Autodesk Inventor part; units mm, degrees
ref_plane "YZ Plane" through (0, 0, 0) normal (1, 0, 0) x (0, 1, 0)
ref_plane "XZ Plane" through (0, 0, 0) normal (0, 1, 0) x (-1, 0, 0)
ref_plane "XY Plane" through (0, 0, 0) normal (0, 0, 1) x (1, 0, 0)
sketch "スケッチ1" plane through (0, 0, 0) normal (0, 0, 1) x (1, 0, 0)
  line L0 (8.5, 7) -> (-8.5, 7)
  line L1 (-8.5, 7) -> (-8.5, -7)
  line L2 (-8.5, -7) -> (8.5, -7)
  line L3 (8.5, -7) -> (8.5, 7)
  line L4 (8.5, 7) -> (-8.5, -7) construction
  line L5 (-8.5, 7) -> (8.5, -7) construction
  circle A0 centre (-6, 0) radius 1.5
  circle A1 centre (6, 0) radius 1.5
  line L6 (-8.5, -6) -> (8.5, -6)
  line L7 (-8.5, 4.5) -> (8.5, 4.5)
  line L8 (-4, -7) -> (-4, 7)
  line L9 (4, -7) -> (4, 7)
  line L10 (2.5, -6) -> (2.5, 4.5)
  line L11 (-2.5, -6) -> (-2.5, 4.5)
  line L12 (1.8, -6) -> (1.8, 4.5)
  line L13 (-1.8, -6) -> (-1.8, 4.5)
  point P0 (0, 0)
  point P1 (-4, -6)
  point P2 (-4, 4.5)
  point P3 (4, -6)
  point P4 (4, 4.5)
  dimension "d0" = 17
  dimension "d1" = 14
  dimension "d2" = 3
  dimension "d3" = 3
  dimension "d4" = 2.5
  dimension "d5" = 4.5
  dimension "d6" = 4.5
  dimension "d7" = 1.5
  dimension "d8" = 1.5
  dimension "d9" = 1
  dimension "d16" = 0.7
  dimension "d17" = 0.7
extrude "押し出し1" add sketch "スケッチ1" along normal blind 7 contours L3 L7 L9 L0 | L9 L7 L8 L0 | L3 L6 L9 L7 | L8 L7 L1 L0 | L3 L2 L9 L6 | L8 L6 L1 L7 | L10 L6 L12 L7 | L9 L2 L8 L6 | L7 L13 L6 L11 | L8 L2 L1 L6
sketch "スケッチ2" plane through (0, 0, 7) normal (0, 0, 1) x (1, 0, 0)
  line L0 (8.5, 7) -> (-8.5, 7)
  line L1 (0, 7) -> (-4, 7)
  line L2 (-4, 7) -> (-4, -7)
  line L3 (-8.5, -7) -> (8.5, -7)
  line L4 (-4, -7) -> (4, -7)
  line L5 (4, -7) -> (4, 7)
  line L6 (4, 7) -> (0, 7)
  point P0 (0, 0)
  dimension "d12" = 4
  dimension "d13" = 8
extrude "押し出し2" cut sketch "スケッチ2" against normal blind 0.6
properties part number "greiper_TPU" material "ゴム、シリコーン"
Model file for the job. Use its own axes, mm. A direction names the side the tool comes from. Coordinates: 2 decimals unless noted, no trailing zeros. Loops run counter-clockwise (first coordinate to the right, second up) from the corner with the lowest first, then second, coordinate; pieces in that order, holes last. Notation, with made-up numbers: (48.5, 6.25) - (95.5, 6.25) arc R31 ccw to (95.5, 37.25) - close; hole circle Ø11 at (-35.5, 2). An arc over 180 degrees is marked (long way). Answer as a JSON object with one key per item and string values. Group by question number.
(1) Cut at D-D (y = -2.5). Give the cut face in (x, z).
(2) Probe line 1 along X through (y, z) = (-3.5, 5.75); line 2 along Y through (x, z) = (-3.5, 5); line 3 along Y through (x, z) = (6, 5.75). List the from-to ranges inside material, lowest first.
(3) Two-plate mould, pull along X, no slides. Class faces 1 (the face through (-3, 4.5, 3)), 2 (the face through (-2.5, -1, 3)), 3 (the face through (-8.5, 0, 3)), 4 (the face through (8, 0, 7)): released by +X, released by -X, zero draft, split by the parting line, or undercut.
(4) Cut at A-A (x = 3.5). Give the cut face in (y, z), then the cut area to 3 significant figures.
(5) Tool access for faces 5 (the face through (0, -6, 3)), 6 (the face through (-2, 2, 6.4)), 7 (the face through (-8, 0, 7)): list every direction of +Z, -Z, +X, -X, +Y, -Y with a clear straight run to the whole face (end or side of a thin tool).
(6) Cut at C-C (z = 5.5). Give the cut face in (x, y), then the cut area to 3 significant figures.
(7) Cut at B-B (y = 0). Give the cut face in (x, z), then the cut area to 3 significant figures.
Geometry says:
{
 "1": {"outline": "(-8.5, 0) - (-4, 0) - (-4, 7) - (-8.5, 7) - close; (-2.5, 0) - (-1.8, 0) - (-1.8, 6.4) - (-2.5, 6.4) - close; (1.8, 0) - (2.5, 0) - (2.5, 6.4) - (1.8, 6.4) - close; (4, 0) - (8.5, 0) - (8.5, 7) - (4, 7) - close"},
 "2": {"line 1": "x = -8.5 to -4, -2.5 to -1.8, 1.8 to 2.5, 4 to 8.5", "line 2": "y = -7 to -6, 4.5 to 7", "line 3": "y = -7 to -1.5, 1.5 to 7"},
 "3": {"face 1": "undercut", "face 2": "undercut", "face 3": "released by -X", "face 4": "zero draft"},
 "4": {"outline": "(-7, 0) - (-6, 0) - (-6, 6.4) - (-7, 6.4) - close; (4.5, 0) - (7, 0) - (7, 6.4) - (4.5, 6.4) - close", "area": "22.4 mm^2"},
 "5": {"face 5": "+Z, -Z", "face 6": "+Z, +Y, -Y", "face 7": "+Z, +X, -X, +Y, -Y"},
 "6": {"outline": "(-8.5, -7) - (8.5, -7) - (8.5, 7) - (-8.5, 7) - close; hole circle Ø3 at (-6, 0); hole (-4, -6) - (-2.5, -6) - (-2.5, 4.5) - (-4, 4.5) - close; hole (-1.8, -6) - (1.8, -6) - (1.8, 4.5) - (-1.8, 4.5) - close; hole (2.5, -6) - (4, -6) - (4, 4.5) - (2.5, 4.5) - close; hole circle Ø3 at (6, 0)", "area": "155 mm^2"},
 "7": {"outline": "(-8.5, 0) - (-7.5, 0) - (-7.5, 7) - (-8.5, 7) - close; (-4.5, 0) - (-4, 0) - (-4, 7) - (-4.5, 7) - close; (-2.5, 0) - (-1.8, 0) - (-1.8, 6.4) - (-2.5, 6.4) - close; (1.8, 0) - (2.5, 0) - (2.5, 6.4) - (1.8, 6.4) - close; (4, 0) - (4.5, 0) - (4.5, 7) - (4, 7) - close; (7.5, 0) - (8.5, 0) - (8.5, 7) - (7.5, 7) - close", "area": "30.0 mm^2"}
}
